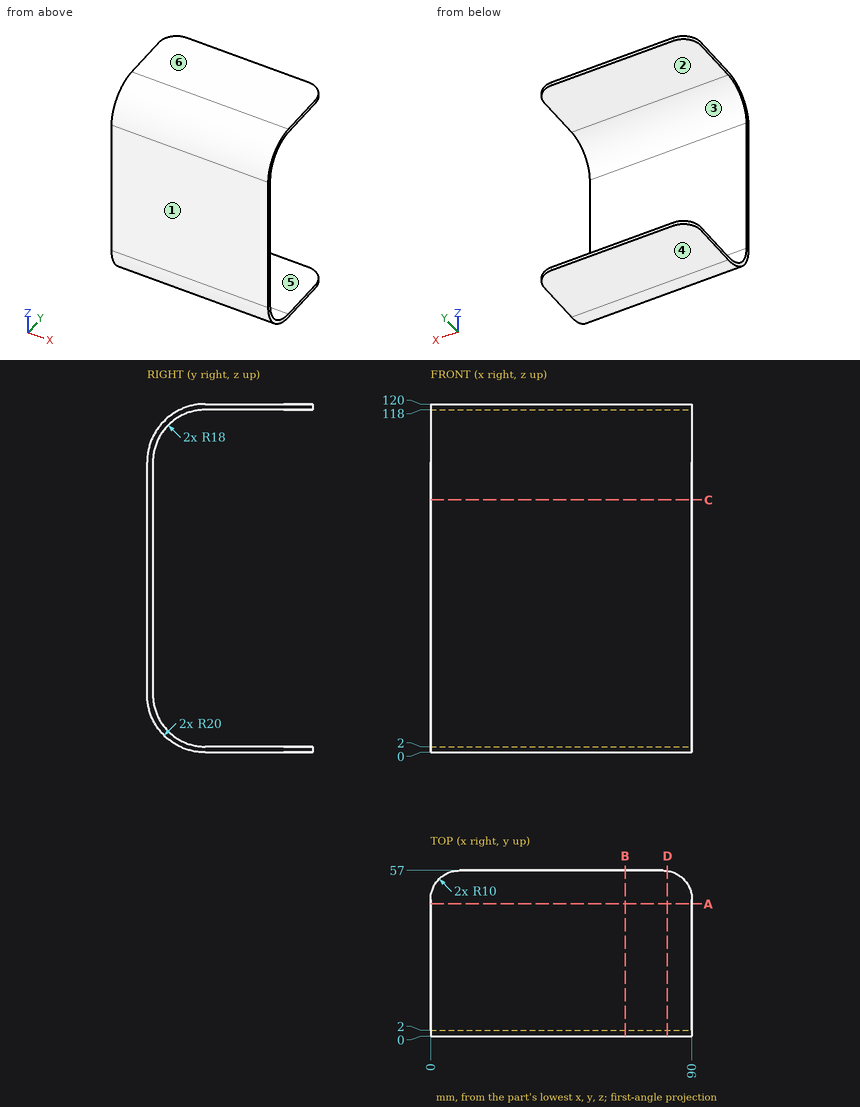
Design review of the part shown in the three views and the two pictorial views. Dimensions are in mm from the part's minimum x, y and z. A direction names the side the tool comes from. Give positions to 0.01 mm unless a question says otherwise; leave off trailing zeros. Write each loop counter-clockwise with the first axis right and the second up, starting at its lowest first coordinate (ties: lowest second). Pieces come first, ordered by that corner, then holes.
Item 1: Wall thickness on probe 1 along Z at (x, y) = (59, 53.5); probe 2 along Y at (x, z) = (21, 87); probe 3 along Z at (x, y) = (9, 16): over which ranges is each line inside the solid? List them lowest first.
Item 2: Take a section at B-B (x = 67). Give the boundary of the cut face in (y, z).
Item 3: Take a section at C-C (z = 87). Give the boundary of the cut face in (x, y).
Item 4: Machinability: for the marked faces 5 and 6, which of the approach directions +Z, -Z, +X, -X, +Y, -Y give a long, thin tool a straight path to every point of the face, cutting with its end or side? Answer none if there is none.
Item 5: Take a section at D-D (x = 81.5). Give the boundary of the cut face in (y, z).
Item 6: Insertion check: P1, Ø3, axis at x = 52, z = 43, coming from the +Y side; P2, Ø6, axis at x = 33.5, y = 16.5, coming from the +Z side. Each pin has a flat end and moves straight along its axis. Give the tip position at first contact, or say it passes through.
Item 7: The part is to be moulded in two halves that separate along Z. For the marked faces 1, 2, 3 and 4, say which applies: +Z half, -Z half, draft (parallel to the pull), parting line (faces both ways), or undercut.
Item 8: Take a section at A-A (y = 45.5). Give the boundary of the cut face in (x, z), and give its area (3 significant figures).
Established:
1. probe 1: z = 0 to 2, 118 to 120
1. probe 2: y = 0 to 2
1. probe 3: z = 0.4 to 2.45, 117.55 to 119.6
2. outline: (0, 20) arc R20 ccw to (20, 0) - (57, 0) - (57, 2) - (20, 2) arc R18 cw to (2, 20) - (2, 100) arc R18 cw to (20, 118) - (57, 118) - (57, 120) - (20, 120) arc R20 ccw to (0, 100) - close
3. outline: (0, 0) - (90, 0) - (90, 2) - (0, 2) - close
4. face 5: +X, -X, +Y
4. face 6: +Z, +X, -X, +Y, -Y
5. outline: (0, 20) arc R20 ccw to (20, 0) - (56.89, 0) - (56.89, 2) - (20, 2) arc R18 cw to (2, 20) - (2, 100) arc R18 cw to (20, 118) - (56.89, 118) - (56.89, 120) - (20, 120) arc R20 ccw to (0, 100) - close
6. P1: stops at y = 2
6. P2: stops at z = 119.99
7. face 1: draft
7. face 2: undercut
7. face 3: undercut
7. face 4: -Z half
8. outline: (0, 0) - (90, 0) - (90, 2) - (0, 2) - close; (0, 118) - (90, 118) - (90, 120) - (0, 120) - close
8. area: 360 mm2
